Job drawing, mm, ordinate dimensions from the low corner. One solid piece. A direction names the side the tool comes from. Give positions to 0.01 mm unless a question says otherwise; leave off trailing zeros. Loops run counter-clockwise (first coordinate to the right, second up) from the corner with the lowest first, then second, coordinate; pieces in that order, holes last. Notation, with made-up numbers: M 41,15 L 88,15 A35 cw 88,47 Z; hole C 72.5,-35.5 d7. An arc over 180 degrees is marked long. Answer in a Markdown table with one row per item.
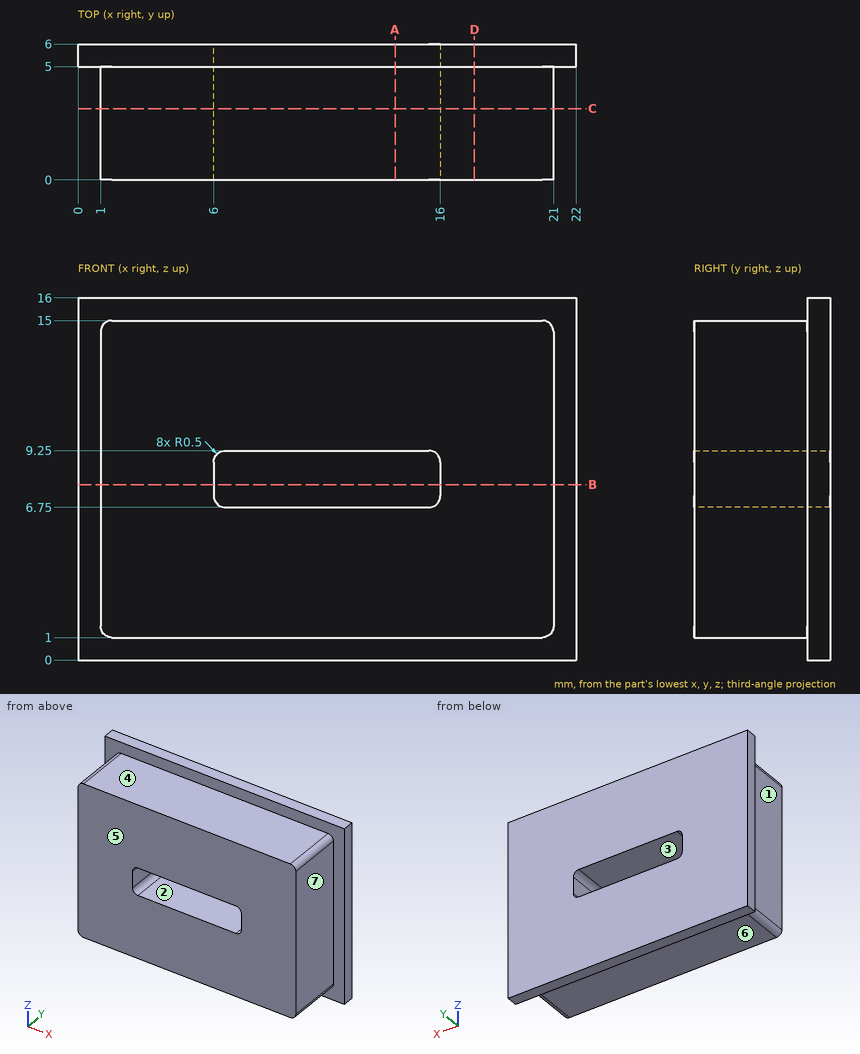
(1) Saw through at A-A (x = 14). Write the cut outline in (y, z), plus the area to 3 significant figures.
Recorded:
| item | result |
|---|---|
| outline | M 0,1 L 5,1 L 5,0 L 6,0 L 6,6.75 L 0,6.75 Z; M 0,9.25 L 6,9.25 L 6,16 L 5,16 L 5,15 L 0,15 Z |
| area | 71.0 mm^2 |
(2) Drill centre lines: line 1 along Z through (x, y) = (9.25, 5.55); line 2 along Z through (x, y) = (7, 0.2); line 3 along Z through (x, y) = (18.5, 3.2). Where is each one in solid material? Low to high.
Recorded:
| item | result |
|---|---|
| line 1 | z = 0 to 6.75, 9.25 to 16 |
| line 2 | z = 1 to 6.75, 9.25 to 15 |
| line 3 | z = 1 to 15 |
(3) Saw through at C-C (y = 3.15). Write the cut outline in (x, z).
Recorded:
| item | result |
|---|---|
| outline | M 1,1.5 A0.5 ccw 1.5,1 L 20.5,1 A0.5 ccw 21,1.5 L 21,14.5 A0.5 ccw 20.5,15 L 1.5,15 A0.5 ccw 1,14.5 Z; hole M 6,7.25 A0.5 ccw 6.5,6.75 L 15.5,6.75 A0.5 ccw 16,7.25 L 16,8.75 A0.5 ccw 15.5,9.25 L 6.5,9.25 A0.5 ccw 6,8.75 Z |
(4) Saw through at D-D (x = 17.5). Write the cut outline in (y, z).
Recorded:
| item | result |
|---|---|
| outline | M 0,1 L 5,1 L 5,0 L 6,0 L 6,16 L 5,16 L 5,15 L 0,15 Z |
(5) Saw through at B-B (z = 7.75). Write the cut outline in (x, y).
Recorded:
| item | result |
|---|---|
| outline | M 0,5 L 1,5 L 1,0 L 6,0 L 6,6 L 0,6 Z; M 16,0 L 21,0 L 21,5 L 22,5 L 22,6 L 16,6 Z |
(6) Which spindle directions (+Z, -Z, +X, -X, +Y, -Y) get a long thin tool onto all of the face, cutting with end or side? Do the marked faces 5, 6 and 7. Say none if no direction does.
Recorded:
| item | result |
|---|---|
| face 5 | +Z, -Z, +X, -X, -Y |
| face 6 | -Z, +X, -X, -Y |
| face 7 | +Z, -Z, +X, -Y |
(7) Pin check, flat tips, straight feed: pin 1 Ø3 at (x, y) = (14, 2) entering from -Z; pin 2 Ø1.5 at (y, z) = (1, 1.5) entering from -X; pin 3 Ø0.8 at (y, z) = (2, 8) entering from +X. Stop position of each tip, or through.
Recorded:
| item | result |
|---|---|
| pin 1 | stops at z = 1 |
| pin 2 | stops at x = 1 |
| pin 3 | stops at x = 21 |
(8) Pull direction Z, two halves, no side cores. Call the marked faces 1, 2, 3 and 4: +Z half, -Z half, draft (parallel to the pull), parting line (faces both ways), or undercut.
Recorded:
| item | result |
|---|---|
| face 1 | draft |
| face 2 | undercut |
| face 3 | undercut |
| face 4 | +Z half |
